```python
from build123d import *

# Parameters (mm, degrees)
SKETCH_1_R          = 7.5
EXTRUDE_1_DEPTH     = 60
SHELL_3_T           = -1.5
SKETCH_4_W          = 25
SKETCH_4_H          = 30
EXTRUDE_4_DEPTH     = 60
SHELL_START         = 61.5
SHELL_4_OUTLINE_W   = 23.5
SHELL_4_OUTLINE_H   = 27
SHELL_4_DEPTH       = 57
SHELL_START_2       = 60
SHELL_4_2_OUTLINE_R = 6
SHELL_4_2_DEPTH     = 1.5
SKETCH_5_R          = 6.2
CUT_EXTRUDE_1_DEPTH = 1.5
SKETCH_18_W         = 18
SKETCH_18_H         = 18
EXTRUDE_10_DEPTH    = 20
SKETCH_19_W         = 15
SKETCH_19_H         = 15
CUT_EXTRUDE_5_DEPTH = 17
SKETCH_20_R         = 6
CUT_EXTRUDE_6_DEPTH = 1.5
SKETCH_22_R         = 7.5
CUT_EXTRUDE_7_DEPTH = 1.5
FILLET_5_R          = 1


# Read off the part's stored shape, not the designer's step: 抽壳4
with BuildPart() as part:
    # 草图1 → 凸台-拉伸1 (new body)
    with BuildSketch(Plane.XY):
        Circle(SKETCH_1_R)
    extrude(amount=EXTRUDE_1_DEPTH)

    # 抽壳3
    shell_3_openings = [part.faces().sort_by_distance(p)[0] for p in [
        (0, 0, 60),
        (0, 0, 0),
    ]]
    offset(amount=SHELL_3_T, openings=shell_3_openings, kind=Kind.INTERSECTION)

    # 草图4 → 凸台-拉伸4 (add)
    with BuildSketch(Plane.XY.offset(60)):
        Rectangle(SKETCH_4_W, SKETCH_4_H)
    extrude(amount=EXTRUDE_4_DEPTH)

    # 抽壳4 outline → 抽壳4 (cut)
    with BuildSketch(Plane.XY.offset(SHELL_START)):
        with Locations((-0.75, 0)):
            Rectangle(SHELL_4_OUTLINE_W, SHELL_4_OUTLINE_H)
    extrude(amount=SHELL_4_DEPTH, mode=Mode.SUBTRACT)

    # Shell 4 2 outline → Shell 4 2 (cut)
    with BuildSketch(Plane.XY.offset(SHELL_START_2)):
        Circle(SHELL_4_2_OUTLINE_R)
    extrude(amount=SHELL_4_2_DEPTH, mode=Mode.SUBTRACT)

    # 草图5 → 切除-拉伸1 (cut)
    with BuildSketch(Plane(origin=(12.5, 0, 0), x_dir=(0, 0, -1), z_dir=(1, 0, 0))):
        with Locations((-90, 0)):
            Circle(SKETCH_5_R)
        with Locations((-107.4, 0)):
            Circle(SKETCH_5_R)
        with Locations(Location((-72.6, 0, 0), (0, 0, 180))):
            Circle(SKETCH_5_R)
    extrude(amount=-CUT_EXTRUDE_1_DEPTH, mode=Mode.SUBTRACT)

    # 草图18 → 凸台-拉伸10 (add)
    with BuildSketch(Plane.XY):
        Rectangle(SKETCH_18_W, SKETCH_18_H)
    extrude(amount=-EXTRUDE_10_DEPTH)

    # 草图19 → 切除-拉伸5 (cut)
    with BuildSketch(Plane.XY.offset(-1.5)):
        Rectangle(SKETCH_19_W, SKETCH_19_H)
    extrude(amount=-CUT_EXTRUDE_5_DEPTH, mode=Mode.SUBTRACT)

    # 草图20 → 切除-拉伸6 (cut)
    with BuildSketch(Plane.XY.offset(-1.5)):
        with Locations(Location((0, 0, 0), (0, 0, 180))):
            Circle(SKETCH_20_R)
    extrude(amount=CUT_EXTRUDE_6_DEPTH, mode=Mode.SUBTRACT)

    # 草图22 → 切除-拉伸7 (cut)
    with BuildSketch(Plane(origin=(0, -9, 0), x_dir=(-1, 0, 0), z_dir=(0, -1, 0))):
        with Locations(Location((0, 10, 0), (0, 0, 90))):
            Circle(SKETCH_22_R)
    extrude(amount=-CUT_EXTRUDE_7_DEPTH, mode=Mode.SUBTRACT)

    # 圆角5
    fillet_5_edges = [part.edges().sort_by_distance(p)[0] for p in [
        (12.5, 0, 60),
        (12.5, -15, 90),
        (0, 15, 60),
        (12.5, 15, 90),
        (0, -15, 60),
        (12.5, 0, 120),
        (0, 15, 120),
        (0, -15, 120),
    ]]
    fillet(fillet_5_edges, radius=FILLET_5_R)


solid = part.part
```
Geometry check sheet. Reference: the model listing, model coordinates, mm. A direction names the side the tool comes from. Give positions to 0.01 mm unless a question says otherwise; leave off trailing zeros. Loops run counter-clockwise (first coordinate to the right, second up) from the corner with the lowest first, then second, coordinate; pieces in that order, holes last. Notation, with made-up numbers: M -6.75,-8 L -1.75,-8 A27 ccw -1.75,17 Z; hole C 18.5,-12 d4. An arc over 180 degrees is marked long. Write item = value, one per line. Start each with the question number.
1. Go/stop test with flat-tipped pins: P1, Ø14.5, axis at x = 1.5, z = -11, coming from the -Y side; P2, Ø6, axis at x = 3.5, z = 30.5, coming from the -Y side; P3, Ø7, axis at x = 1.5, z = -6.5, coming from the +Y side. Record where each tip stops, or that it passes through.
2. Tool access check on faces 1 (the face through (-1, 0, 118.5)), 2 (the face through (0, 7.5, -10)), 3 (the face through (-1, 15, 90)), 4 (the face through (0, 9, -10)), 5 (the face through (0, 0, -20)). Record the directions out of +Z, -Z, +X, -X, +Y, -Y that give a thin tool (end or side, any length) a straight path to the whole face; none if there is none.
3. Thickness scan on probe 1 along Z at (x, y) = (0, -8.05); probe 2 along Z at (x, y) = (-7, 0); probe 3 along Y at (x, z) = (0, 43). Record the ranges inside material, lowest first.
4. Section check D-D, the plane y = 0. Give the number of separate pieces and of enclosed holes in the cut face, plus the area to 3 significant figures.
5. Draft check along Y on faces 6 (the face through (-1, 13.5, 90)), 7 (the face through (-9, 0, -10)), 8 (the face through (-6, -9, -5)), 9 (the face through (1, -7.5, -2)). Enter one of: +Y half, -Y half, draft (parallel to the pull), parting line (faces both ways), or undercut.
6. Section check C-C, the plane z = 33.5. Enter the section's corners in (x, y).
7. Section check A-A, the plane z = 71. Enter the section's corners in (x, y), plus the area to 3 significant figures.
Values follow:
q1.P1 = -9
q1.P2 = -7.48
q1.P3 = 9
q2.face_1 = -X
q2.face_2 = none
q2.face_3 = +Z, -Z, +X, -X, +Y
q2.face_4 = -Z, +X, -X, +Y
q2.face_5 = -Z, +X, -X, +Y, -Y
q3.probe_1 = -20 to -17.5, -2.5 to 0, 60 to 61.5, 118.5 to 120
q3.probe_2 = -20 to -18.5, -1.5 to 61.5, 118.5 to 120
q3.probe_3 = -7.5 to -6, 6 to 7.5
q4.separate_pieces = 4
q4.enclosed_holes = 0
q4.area = 353 mm^2
q5.face_6 = undercut
q5.face_7 = draft
q5.face_8 = -Y half
q5.face_9 = undercut
q6.outline = C 0,0 d15; hole C 0,0 d12
q7.outline = M -12.5,-15 L 11.5,-15 A1 ccw 12.5,-14 L 12.5,-5.99 L 11,-5.99 L 11,-13.5 L -12.5,-13.5 Z; M -12.5,13.5 L 11,13.5 L 11,5.99 L 12.5,5.99 L 12.5,14 A1 ccw 11.5,15 L -12.5,15 Z
q7.area = 97.1 mm^2
